Here's how the part is built. I have some questions about the finished solid (model axes, mm). A direction names the side the tool comes from. Give positions to 0.01 mm unless a question says otherwise; leave off trailing zeros. Answer as CSV lines item,"result". Start each with the question number.
Item 1: If we mould it in two halves opening along Z, with no side actions, what happens to faces 1 (the cylindrical face through (-4.348, 1.521, 2.468)), 2 (the flat face through (-6, 1.5, 23))? For each: released by +Z, released by -Z, zero draft, split by the parting line, or undercut.
Item 2: If I drill on line 1 along Z through (x, y) = (0, 0.8); line 2 along Z through (x, y) = (2, 0.7); line 3 along X through (y, z) = (1.1, -15.5), over which ranges is the centre line in solid material (lowest first)? Write a range as from..to.
Item 3: Will these pins go through, and if not, where does the flat tip stop? P1, Ø3.5, axis at x = 0, z = 0, coming from the -Y side; P2, Ø5, axis at x = 17.5, z = 20, coming from the -Y side; P3, Ø1, axis at x = -11, z = -11.5, coming from the -Y side; P4, Ø0.6, axis at x = 6.5, y = 1.5, coming from the +Z side.
Item 4: For faces 3 (the flat face through (4.993, 1.521, -8.648)), 4 (the flat face through (0, 0, 6)), which set-ups out of +Z, -Z, +X, -X, +Y, -Y let a thin tool reach every point of the face, with its end or its side?
Item 5: I want a section at A-A on x = 0. Give the number of separate pieces and of enclosed holes in the cut face, plus the area to 3 significant figures.
Autodesk Inventor part; units mm, degrees
ref_plane "YZ Plane" through (0, 0, 0) normal (1, 0, 0) x (0, 1, 0)
ref_plane "XZ Plane" through (0, 0, 0) normal (0, 1, 0) x (-1, 0, 0)
ref_plane "XY Plane" through (0, 0, 0) normal (0, 0, 1) x (1, 0, 0)
sketch "Náčrt1" plane through (0, 0, 0) normal (0, 1, 0) x (-1, 0, 0)
  line L0 (0, -38.2576) -> (0, 38.2576)
  line L1 (-38.2576, 0) -> (38.2576, 0)
  circle A0 centre (0, 0) radius 23.55
  dimension "d0" = 47.1
extrude "Vysunutí1" add sketch "Náčrt1" along normal blind 1.5
sketch "Náčrt2" plane through (0, 1.5, 0) normal (0, 1, 0) x (1, 0, 0)
  line L0 (0, 36.47) -> (0, -36.47)
  line L1 (36.47, 0) -> (-36.47, 0)
  circle A0 centre (0, 0) radius 26.05
  dimension "d3" = 52.1
extrude "Vysunutí2" add sketch "Náčrt2" along normal blind 1.5
chamfer "Zkosení1" distance 1.5 angle 45 1 edges at (-26.05, 3, 0)
sketch "Náčrt3" plane through (0, 3, 0) normal (0, 1, 0) x (1, 0, 0)
  line L0 (0, 36.47) -> (0, -36.47)
  line L1 (36.47, 0) -> (-36.47, 0)
  arc A0 (2.5, 4.3301) -> (-2.5, 4.3301) centre (0, 0) ccw
  arc A1 (3.5, 6.0622) -> (-3.5, 6.0622) centre (0, 0) ccw
  line L2 (-2.5, 4.3301) -> (-3.5, 6.0622)
  line L3 (2.5, 4.3301) -> (3.5, 6.0622)
  arc A2 (4.5, 7.7942) -> (-4.5, 7.7942) centre (0, 0) ccw
  arc A3 (5.5, 9.5263) -> (-5.5, 9.5263) centre (0, 0) ccw
  line L4 (-4.5, 7.7942) -> (-5.5, 9.5263)
  line L5 (4.5, 7.7942) -> (5.5, 9.5263)
  arc A4 (6.5, 11.2583) -> (-6.5, 11.2583) centre (0, 0) ccw
  arc A5 (7.5, 12.9904) -> (-7.5, 12.9904) centre (0, 0) ccw
  line L6 (-6.5, 11.2583) -> (-7.5, 12.9904)
  line L7 (6.5, 11.2583) -> (7.5, 12.9904)
  arc A6 (8.5, 14.7224) -> (-8.5, 14.7224) centre (0, 0) ccw
  arc A7 (9.5, 16.4545) -> (-9.5, 16.4545) centre (0, 0) ccw
  line L8 (-8.5, 14.7224) -> (-9.5, 16.4545)
  line L9 (8.5, 14.7224) -> (9.5, 16.4545)
  dimension "d10" = 5
  dimension "d11" = 7
  dimension "d12" = 60
  dimension "d24" = 9
  dimension "d25" = 11
  dimension "d26" = 13
  dimension "d27" = 15
  dimension "d28" = 17
  dimension "d29" = 19
extrude "Vysunutí3" cut sketch "Náčrt3" against normal through all
pattern_circular "Kruhové pole1" count 3 over 360 about axis through (0, -10, 0) along (0, 1, 0) of "Vysunutí3"
sketch "Náčrt4" plane through (0, 3, 0) normal (0, 1, 0) x (1, 0, 0)
  line L0 (0, 36.47) -> (0, -36.47)
  line L1 (36.47, 0) -> (-36.47, 0)
  circle A0 centre (0, 0) radius 3
  dimension "d18" = 6
extrude "Vysunutí4" cut sketch "Náčrt4" against normal through all
properties part number "4.L - GM - 01.04" material "LCP plast"
Result:
1,face 1,"undercut"
1,face 2,"zero draft"
2,line 1,"-23.55..-19, -17..-15, -13..-11, -9..-7, -5..-3, 3..23.55"
2,line 2,"-23.46..-18.89, -16.88..-14.87, -12.85..-10.82, -8.77..-6.71, -4.58..-2.24, 2.24..23.46"
2,line 3,"-17.73..-8.95, -6.98..6.98, 8.95..17.73"
3,P1,"through"
3,P2,"y = 1.5"
3,P3,"y = 0"
3,P4,"z = 25.3"
4,face 3,"+Y, -Y"
4,face 4,"+Z, -Z, +X, -X, -Y"
5,separate pieces,"6"
5,enclosed holes,"0"
5,area,"105 mm^2"
